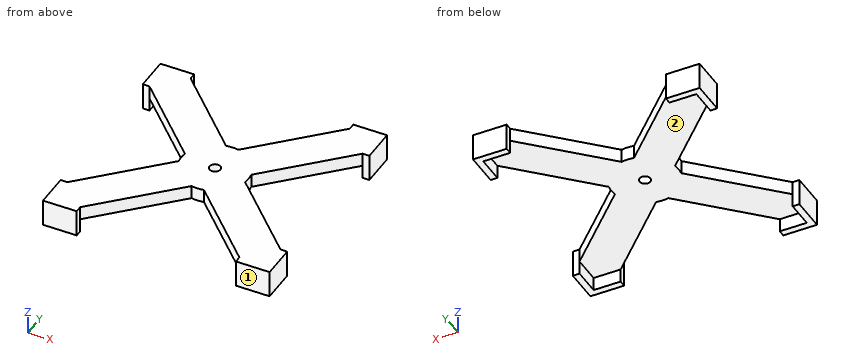
```python
from build123d import *

# Parameters (mm, degrees)
CROQUIS1_R              = 4
SALIENTE_EXTRUIR1_DEPTH = 10
SALIENTE_EXTRUIR2_DEPTH = 20


with BuildPart() as part:
    # Croquis1 → Saliente-Extruir1 (new body)
    with BuildSketch(Plane.XY):
        with BuildLine():
            Line((-59, 78.65), (-4.600099172, 24.573137521))
            ThreePointArc((-4.600099172, 24.573137521), (0, 25), (4.600099172, 24.573137521))
            Line((4.600099172, 24.573137521), (59, 78.65))
            Line((59, 78.65), (79, 78.65))
            Line((79, 78.65), (79, 58.530526224))
            Line((79, 58.530526224), (24.600099172, 4.453663744))
            ThreePointArc((24.600099172, 4.453663744), (25, 0), (24.600099172, -4.453663744))
            Line((24.600099172, -4.453663744), (79, -58.530526224))
            Line((79, -58.530526224), (79, -78.65))
            Line((79, -78.65), (59, -78.65))
            Line((59, -78.65), (4.600099172, -24.573137521))
            ThreePointArc((4.600099172, -24.573137521), (0, -25), (-4.600099172, -24.573137521))
            Line((-4.600099172, -24.573137521), (-59, -78.65))
            Line((-59, -78.65), (-79, -78.65))
            Line((-79, -78.65), (-79, -58.530526224))
            Line((-79, -58.530526224), (-24.600099172, -4.453663744))
            ThreePointArc((-24.600099172, -4.453663744), (-25, 0), (-24.600099172, 4.453663744))
            Line((-24.600099172, 4.453663744), (-79, 58.530526224))
            Line((-79, 58.530526224), (-79, 78.65))
            Line((-79, 78.65), (-59, 78.65))
        make_face()
        Circle(CROQUIS1_R, mode=Mode.SUBTRACT)
    extrude(amount=SALIENTE_EXTRUIR1_DEPTH)

    # Croquis4 → Saliente-Extruir2 (add)
    with BuildSketch(Plane.XY.offset(10)):
        Polygon((-59, 78.65), (-79, 78.65), (-79, 58.530526224), (-84, 58.530526224), (-84, 83.65), (-79, 83.65), (-59, 83.65), align=None)
        Polygon((59, 78.65), (59, 83.65), (79, 83.65), (84, 83.65), (84, 58.530526224), (79, 58.530526224), (79, 78.65), align=None)
        Polygon((59, -78.65), (79, -78.65), (79, -58.530526224), (84, -58.530526224), (84, -83.65), (79, -83.65), (59, -83.65), align=None)
        Polygon((-59, -78.65), (-59, -83.65), (-79, -83.65), (-84, -83.65), (-84, -58.530526224), (-79, -58.530526224), (-79, -78.65), align=None)
    extrude(amount=-SALIENTE_EXTRUIR2_DEPTH)


solid = part.part
```
CAD build for the part. Positions are in the model's coordinates, mm. Face numbers are marked on the shaded views. Round coordinates to 2 decimals unless told otherwise and drop trailing zeros. Write each loop counter-clockwise with the first axis right and the second up, starting at its lowest first coordinate (ties: lowest second). Pieces come first, ordered by that corner, then holes. Notation, with made-up numbers: (29.25, 55) - (75.25, 55) arc R12 cw to (75.25, 73) - close; hole circle Ø8 at (-16.75, -4). An arc over 180 degrees is marked (long way). Return JSON: item names as keys, results as strings. Group by question number.
Item 1: Mould opens along X. For the marked faces 1 and 2 say: +X half, -X half, draft (parallel to the pull), parting line (faces both ways), or undercut.
Item 2: Probe probe 1 along Y at (x, z) = (0, 2); probe 2 along Y at (x, z) = (-62.5, -6); probe 3 along X at (y, z) = (74, -2). List the from-to ranges inside material, lowest first.
Item 3: Band-saw the part on A-A on y = 0. List the corners of the cut face in (x, z), plus the area to 3 significant figures.
Item 4: Flat gauge pins, fed straight in: pin 1 Ø8 at (y, z) = (55, 6) entering from -X; pin 2 Ø10 at (y, z) = (-4.5, -1.5) entering from -X; pin 3 Ø3 at (y, z) = (-55, 3.5) entering from -X; pin 4 Ø2 at (y, z) = (27.5, 7) entering from +X. Where does each tip first touch, or does it go through?
Item 5: Band-saw the part on B-B on z = -7.25. List the corners of the cut face in (x, y), plus the area to 3 significant figures.
Resolved:
{
 "1": {"face 1": "draft", "face 2": "undercut"},
 "2": {"probe 1": "y = -25 to -4, 4 to 25", "probe 2": "y = -83.65 to -78.65, 78.65 to 83.65", "probe 3": "x = -84 to -79, 79 to 84"},
 "3": {"outline": "(-25, 0) - (-4, 0) - (-4, 10) - (-25, 10) - close; (4, 0) - (25, 0) - (25, 10) - (4, 10) - close", "area": "420 mm²"},
 "4": {"pin 1": "stops at x = -84", "pin 2": "stops at x = -29.44", "pin 3": "stops at x = -76.96", "pin 4": "stops at x = 48.79"},
 "5": {"outline": "(-84, -83.65) - (-59, -83.65) - (-59, -78.65) - (-79, -78.65) - (-79, -58.53) - (-84, -58.53) - close; (-84, 58.53) - (-79, 58.53) - (-79, 78.65) - (-59, 78.65) - (-59, 83.65) - (-84, 83.65) - close; (59, -83.65) - (84, -83.65) - (84, -58.53) - (79, -58.53) - (79, -78.65) - (59, -78.65) - close; (59, 78.65) - (79, 78.65) - (79, 58.53) - (84, 58.53) - (84, 83.65) - (59, 83.65) - close", "area": "902 mm²"}
}
